Source: three-view drawing plus pictorial views. Frame: mm from the lowest corner of the part. A direction names the side the tool comes from. Give positions to 0.01 mm unless a question says otherwise; leave off trailing zeros. Write each loop counter-clockwise with the first axis right and the second up, starting at its lowest first coordinate (ties: lowest second). Pieces come first, ordered by that corner, then holes.
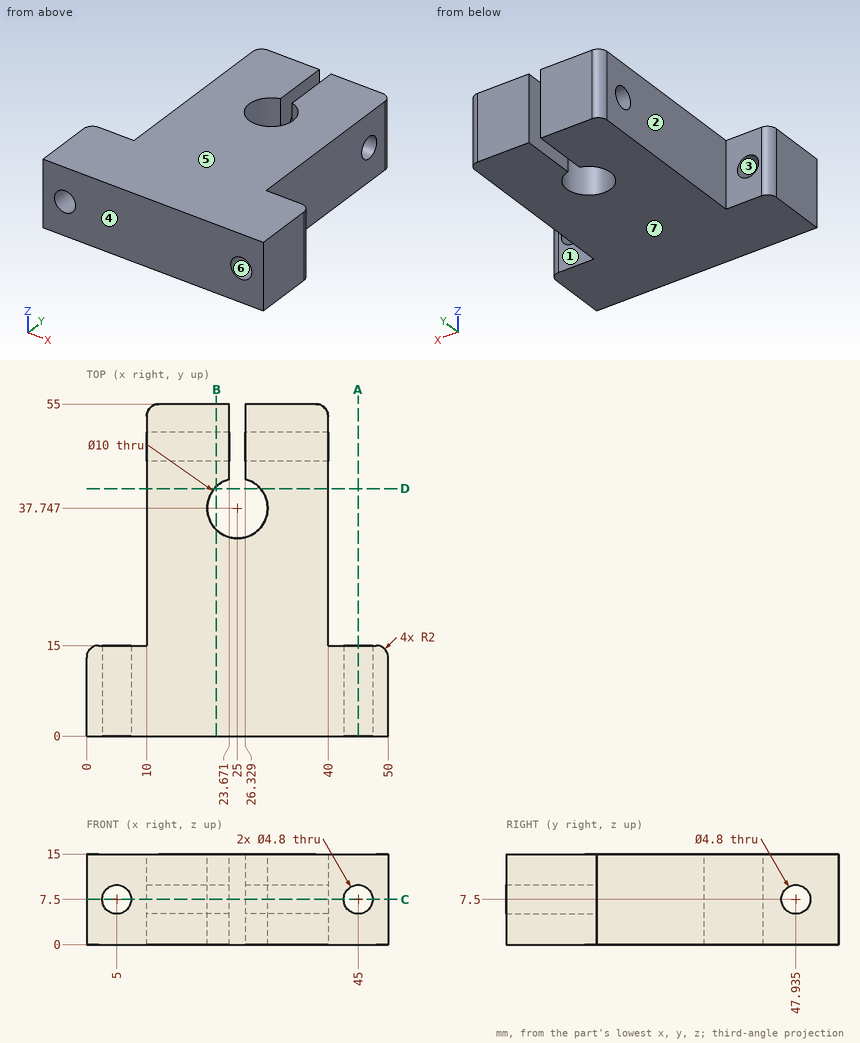
Q1. Access query for the marked faces 1, 2 and 3. Directions: +Z, -Z, +X, -X, +Y, -Y. A direction counts if a zero-diameter tool reaches every point of the face in a straight line with its end or side. Return the directions, or none.
Filled sheet:
face 1: +Z, -Z, +X, +Y
face 2: +Z, -Z, -X, +Y
face 3: +Y, -Y
Q2. Pin query (flat end, axial travel): P1, Ø6.5, axis at x = 42.5, z = 11, coming from the +Y side; P2, Ø6, axis at y = 49, z = 7.5, coming from the +X side; P3, Ø9, axis at x = 4.5, z = 9.5, coming from the +Y side. Return the tip coordinate at first contact, or that it passes through.
Filled sheet:
P1: stops at y = 54.56
P2: stops at x = 40
P3: stops at y = 15
Q3. Pull-direction query (Z, two-part tool) for the marked faces 4, 5, 6 and 7; classes: released by +Z, released by -Z, zero draft, split by the parting line, or undercut.
Filled sheet:
face 4: zero draft
face 5: released by +Z
face 6: undercut
face 7: released by -Z
Q4. Section D-D on y = 41. Output: boundary loops of the cut face in (x, z), plus the area to 3 significant figures.
Filled sheet:
outline: (10, 0) - (21.2, 0) - (21.2, 15) - (10, 15) - close; (28.8, 0) - (40, 0) - (40, 15) - (28.8, 15) - close
area: 336 mm2
Q5. Section C-C on z = 7.5. Count the separate pieces of the cut face and the enclosed holes in it, plus the area to 3 significant figures.
Filled sheet:
separate pieces: 5
enclosed holes: 0
area: 1,560 mm2
Q6. Section B-B on x = 21.5. Output: boundary loops of the cut face in (y, z) (1 decimal), plus the area to 3 significant figures.
Filled sheet:
outline: (0, 0) - (34.2, 0) - (34.2, 15) - (0, 15) - close; (41.3, 0) - (55, 0) - (55, 15) - (41.3, 15) - close; hole circle Ø4.8 at (47.9, 7.5)
area: 700 mm2
Q7. Ray query, line 1 along X through (y, z) = (10.75, 7.5); line 2 along X through (y, z) = (52, 10.5); line 3 along Y through (x, z) = (12.5, 7.75). Return the intervals inside material, ascending.
Filled sheet:
line 1: x = 0 to 2.6, 7.4 to 42.6, 47.4 to 50
line 2: x = 10 to 23.67, 26.33 to 40
line 3: y = 0 to 45.55, 50.32 to 55
Q8. Section A-A on x = 45. Output: boundary loops of the cut face in (y, z), plus the area to 3 significant figures.
Filled sheet:
outline: (0, 0) - (15, 0) - (15, 5.1) - (0, 5.1) - close; (0, 9.9) - (15, 9.9) - (15, 15) - (0, 15) - close
area: 153 mm2
